Verification items for this drawing (mm, ordinates from the low corner). Coordinates: 2 decimals unless noted, no trailing zeros. Write each loop counter-clockwise with the first axis right and the second up, starting at its lowest first coordinate (ties: lowest second). Pieces come first, ordered by that corner, then holes. Notation, with made-up numbers: (-29.75, 12.5) -> (29.25, 12.5) arc R22 cw to (29.25, 22.5) -> close; hole circle Ø10 at (-26.75, -28.5). An arc over 180 degrees is marked (long way). Answer as CSV lines item,"result".
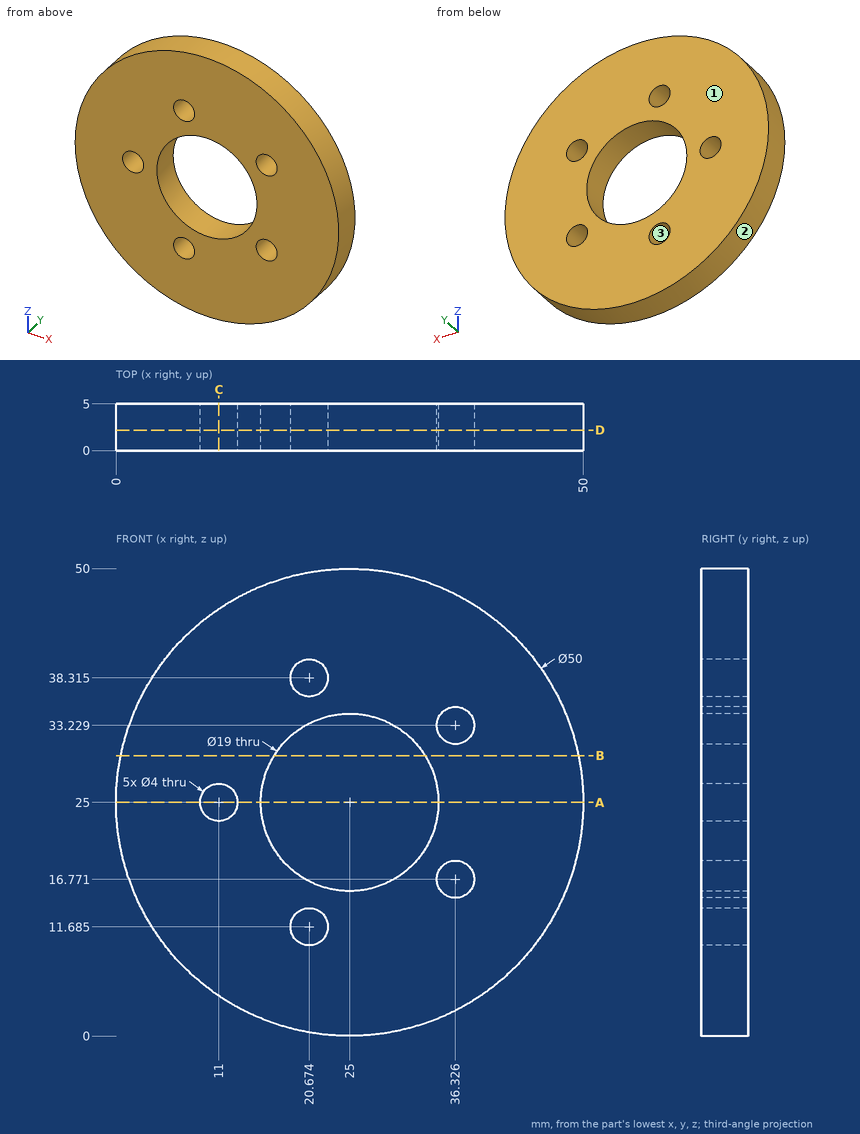
Item 1: Cross-section at A-A, the plane z = 25. Record the cut outline in (x, y), plus the area to 3 significant figures.
Responses:
outline,"(0, 0) -> (9, 0) -> (9, 5) -> (0, 5) -> close; (13, 0) -> (15.5, 0) -> (15.5, 5) -> (13, 5) -> close; (34.5, 0) -> (50, 0) -> (50, 5) -> (34.5, 5) -> close"
area,"135 mm2"
Item 2: Depth check by flat-ended pin: pin 1 Ø3 at (y, z) = (4.5, 19) entering from -X; pin 2 Ø2.5 at (x, z) = (11, 25) entering from +Y; pin 3 Ø1.5 at (x, y) = (19.5, 0.5) entering from +Z; pin 4 Ø1 at (x, y) = (24.5, 2) entering from +Z. Enter the tip coordinate at first touch or a pass-through.
Responses:
pin 1,"stops at x = 0.41"
pin 2,"passes through"
pin 3,"stops at z = 49.54"
pin 4,"stops at z = 50"
Item 3: Cross-section at C-C, the plane x = 11. Record the cut outline in (y, z).
Responses:
outline,"(0, 4.29) -> (5, 4.29) -> (5, 23) -> (0, 23) -> close; (0, 27) -> (5, 27) -> (5, 45.71) -> (0, 45.71) -> close"
Item 4: Release check for a two-part mould opening along Z. For the marked faces 1, 2 and 3 record: +Z half, -Z half, draft (parallel to the pull), parting line (faces both ways), or undercut.
Responses:
face 1,"draft"
face 2,"parting line"
face 3,"undercut"
Item 5: Thickness scan on probe 1 along Z at (x, y) = (19, 3.1) (1 decimal); probe 2 along X at (y, z) = (2.35, 16.5) (1 decimal); probe 3 along Z at (x, y) = (25.5, 0.55) (1 decimal). Record the ranges inside material, lowest first.
Responses:
probe 1,"z = 0.7 to 10.6, 12.8 to 17.6, 32.4 to 37.2, 39.4 to 49.3"
probe 2,"x = 1.5 to 20.8, 29.2 to 34.3, 38.3 to 48.5"
probe 3,"z = 0 to 15.5, 34.5 to 50"
Item 6: Cross-section at D-D, the plane y = 2.2. Record the cut outline in (x, z) (1 decimal).
Responses:
outline,"circle Ø50 at (25, 25); hole circle Ø4 at (11, 25); hole circle Ø19 at (25, 25); hole circle Ø4 at (20.7, 11.7); hole circle Ø4 at (20.7, 38.3); hole circle Ø4 at (36.3, 16.8); hole circle Ø4 at (36.3, 33.2)"
Item 7: Cross-section at B-B, the plane z = 30. Record the cut outline in (x, y) (1 decimal), plus the area to 3 significant figures.
Responses:
outline,"(0.5, 0) -> (16.9, 0) -> (16.9, 5) -> (0.5, 5) -> close; (33.1, 0) -> (49.5, 0) -> (49.5, 5) -> (33.1, 5) -> close"
area,"164 mm2"
